```python
from build123d import *

# Parameters (mm, degrees)
F2_W          = 304.8
F2_H          = 304.8
F3_DEPTH      = 6.35
F5_R          = 36.5125
F5_R_2        = 30.1625
F6_DEPTH      = 292.1
F6_DEPTH_BACK = 15.24
F8_DEPTH      = 50.8
F8_DEPTH_BACK = 50.8
F9_R          = 4.7625
F10_DEPTH     = 1.27
F11_R         = 6.35
F12_DEPTH     = 25.4


with BuildPart() as f3:
    # F2 (on line) → F3 (new body)
    with BuildSketch(Plane(origin=(0, 0, 0), x_dir=(1, 0, 0), z_dir=(0, 0.1736481777, 0.984807753))):
        with Locations((-12.7, 0)):
            Rectangle(F2_W, F2_H)
    extrude(amount=F3_DEPTH)

    # F5 (on line) → F6 (join, two sides)
    with BuildSketch(Plane(origin=(0, 0, 0), x_dir=(0.8660254038, 0, -0.5), z_dir=(-0.5, 0, -0.8660254038))) as f6_sk:
        Circle(F5_R)
        Circle(F5_R_2, mode=Mode.SUBTRACT)
    extrude(amount=-F6_DEPTH)
    extrude(f6_sk.sketch, amount=F6_DEPTH_BACK)

    # F7 (on Right) → F8 (cut, two sides)
    with BuildSketch(Plane.YZ) as f8_sk:
        Polygon((47.014611039, -36.6175852823), (47.014611039, -8.2899444137), (-48.9987151589, 8.6397955026), (-48.9987151589, -36.6175852823), align=None)
    extrude(amount=-F8_DEPTH, mode=Mode.SUBTRACT)
    extrude(f8_sk.sketch, amount=F8_DEPTH_BACK, mode=Mode.SUBTRACT)

    # F9 (on face) → F10 (cut)
    with BuildSketch(Plane(origin=(0, 1.1026659282, 6.2535292316), x_dir=(1, 0, 0), z_dir=(0, 0.1736481777, 0.984807753))):
        with Locations((114.3, 0)):
            Circle(F9_R)
        with Locations((-12.7, -76.2)):
            Circle(F9_R)
        with Locations((63.5, 0)):
            Circle(F9_R)
        with Locations((-12.7, -127)):
            Circle(F9_R)
    extrude(amount=-F10_DEPTH, mode=Mode.SUBTRACT)

    # F11 (on face) → F12 (cut)
    with BuildSketch(Plane(origin=(0, 1.1026659282, 6.2535292316), x_dir=(1, 0, 0), z_dir=(0, 0.1736481777, 0.984807753))):
        with Locations((-139.7, 127)):
            Circle(F11_R)
        with Locations((114.3, 127)):
            Circle(F11_R)
        with Locations((114.3, -127)):
            Circle(F11_R)
        with Locations((-139.7, -127)):
            Circle(F11_R)
    extrude(amount=-F12_DEPTH, mode=Mode.SUBTRACT)


solid = f3.part
```
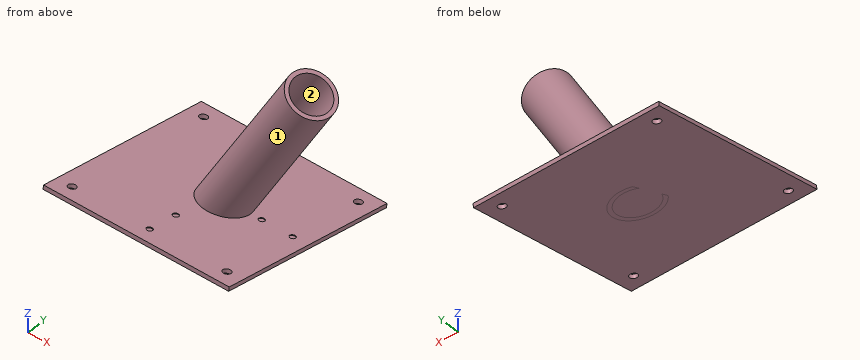
The model under review builds one solid part; all positions refer to its coordinate system, in mm. Face numbers are marked on the shaded views. Round coordinates to 2 decimals unless told otherwise and drop trailing zeros. Order: outer loops, then holes, each group sorted by start corner. A loop starts at its lowest first (then second) coordinate and runs counter-clockwise, first axis right, second up. Notation, with made-up numbers: (57, -11.5) - (91, -11.5) arc R29 cw to (91, 24.5) - close; hole circle Ø6 at (-37.75, 84). An arc over 180 degrees is marked (long way). Answer in a Markdown table with one row per item.
(1) Clearance check with flat-ended pins moving along their axes: P1, Ø3, axis at x = 75.5, z = 74.5, coming from the +Y side; P2, Ø8, axis at x = 79, z = 204.5, coming from the -Y side; P3, Ø4, axis at x = -44, y = 114.5, coming from the +Z side. State where each tip first meets the part, or that it passes through.
Result set:
| item | result |
|---|---|
| P1 | stops at y = 24.97 |
| P2 | stops at y = -21.05 |
| P3 | stops at z = -13.39 |
(2) For line 1 (X direction, y = 13.5, z = 207); line 2 (Y direction, x = -1.5, z = 52.5); line 3 (Y direction, x = 103.5, z = 191), list the stretches that pass through material, from the lowest coordinate up. Write a range as from..to.
Result set:
| item | result |
|---|---|
| line 1 | x = 80.34..88.37, 150.66..158.68 |
| line 2 | y = -23.96..-12.28, 12.28..23.96 |
| line 3 | y = -36.04..-29.59, 29.59..36.04 |
(3) Take a section at B-B on y = -64. Write out the cut boundary in (x, z), plus the area to 3 significant figures.
Result set:
| item | result |
|---|---|
| outline | (-165.1, 11.28) - (139.7, 11.28) - (139.7, 17.73) - (-165.1, 17.73) - close |
| area | 1,970 mm2 |
(4) Take a section at A-A on x = -102.5. Write out the cut boundary in (y, z).
Result set:
| item | result |
|---|---|
| outline | (-150.08, 26.46) - (150.08, -26.46) - (151.19, -20.21) - (-148.98, 32.72) - close |
(5) Mouldability with a two-part tool opening along Z and no side actions: class the marked faces 1 and 2 as released by +Z, released by -Z, zero draft, split by the parting line, or undercut.
Result set:
| item | result |
|---|---|
| face 1 | undercut |
| face 2 | undercut |
(6) Take a section at C-C on x = 99. Count the separate pieces of the cut face and the enclosed holes in it, plus the area to 3 significant figures.
Result set:
| item | result |
|---|---|
| separate pieces | 2 |
| enclosed holes | 1 |
| area | 4,600 mm2 |
